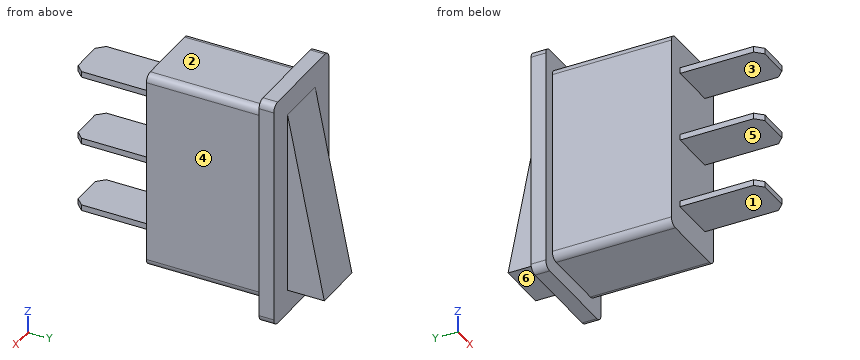
from build123d import *

# Parameters (mm, degrees)
SKIZZE1_W                            = 14
SKIZZE1_H                            = 31.5
AUFSATZ_LINEAR_AUSTRAGEN1_DEPTH      = 2
VERRUNDUNG1_R                        = 1
SKIZZE2_W                            = 10.7
SKIZZE2_H                            = 27.2
AUFSATZ_LINEAR_AUSTRAGEN2_DEPTH      = 16.2
VERRUNDUNG2_R                        = 1
SKIZZE3_W                            = 6.3
SKIZZE3_H                            = 0.8
AUFSATZ_LINEAR_AUSTRAGEN3_DEPTH      = 11
LINEARES_MUSTER1_COUNT               = 2
LINEARES_MUSTER1_PITCH               = 9.5
LINEARES_MUSTER1_COL_COUNT           = 2
LINEARES_MUSTER1_COL_PITCH           = 9.5
SCHNITT_LINEAR_AUSTRAGEN1_DEPTH      = 40.921955112
AUFSATZ_LINEAR_AUSTRAGEN4_DEPTH      = 3.5
AUFSATZ_LINEAR_AUSTRAGEN4_DEPTH_BACK = 3.5


with BuildPart() as part:
    # Skizze1 → Aufsatz-Linear austragen1 (new body)
    with BuildSketch(Plane(origin=(0, 0, 0), x_dir=(1, 0, 0), z_dir=(0, 1, 0))):
        with Locations((7, 15.75)):
            Rectangle(SKIZZE1_W, SKIZZE1_H)
    extrude(amount=AUFSATZ_LINEAR_AUSTRAGEN1_DEPTH)

    # Verrundung1
    verrundung1_edges = [part.edges().sort_by_distance(p)[0] for p in [
        (0, 1, -31.5),
        (14, 1, -31.5),
        (14, 1, 0),
        (0, 1, 0),
    ]]
    fillet(verrundung1_edges, radius=VERRUNDUNG1_R)

    # Skizze2 → Aufsatz-Linear austragen2 (add)
    with BuildSketch(Plane.XZ):
        with Locations((7, -15.75)):
            Rectangle(SKIZZE2_W, SKIZZE2_H)
    extrude(amount=AUFSATZ_LINEAR_AUSTRAGEN2_DEPTH)

    # Verrundung2
    verrundung2_edges = [part.edges().sort_by_distance(p)[0] for p in [
        (12.35, -8.1, -29.35),
        (12.35, -8.1, -2.15),
        (1.65, -8.1, -2.15),
        (1.65, -8.1, -29.35),
    ]]
    fillet(verrundung2_edges, radius=VERRUNDUNG2_R)

    # Skizze3 → Aufsatz-Linear austragen3 (add)
    with BuildSketch(Plane.XZ.offset(16.2)):
        with Locations((7, -15.75)):
            Rectangle(SKIZZE3_W, SKIZZE3_H)
    aufsatz_linear_austragen3 = extrude(amount=AUFSATZ_LINEAR_AUSTRAGEN3_DEPTH)

    # Lineares Muster1: Aufsatz-Linear austragen3 ×2
    with Locations(*[(0, 0, -i * LINEARES_MUSTER1_PITCH) for i in range(1, LINEARES_MUSTER1_COUNT)]):
        add(aufsatz_linear_austragen3)

    # Lineares Muster1 col: Aufsatz-Linear austragen3 ×2
    with Locations(*[(0, 0, i * LINEARES_MUSTER1_COL_PITCH) for i in range(1, LINEARES_MUSTER1_COL_COUNT)]):
        add(aufsatz_linear_austragen3)

    # Skizze4 → Schnitt-Linear austragen1 (cut, through all)
    with BuildSketch(Plane.XY.offset(-5.85)):
        Polygon((3.85, -26.2), (3.85, -27.2), (4.85, -27.2), align=None)
        Polygon((9.15, -27.2), (10.15, -26.2), (10.15, -27.2), align=None)
    extrude(amount=-SCHNITT_LINEAR_AUSTRAGEN1_DEPTH, mode=Mode.SUBTRACT)

    # Skizze5 → Aufsatz-Linear austragen4 (add, two sides: drawn at the far end of the back side and taken through both)
    with BuildSketch(Plane(origin=(7, 0, 0), x_dir=(0, 0, -1), z_dir=(1, 0, 0)).offset(-AUFSATZ_LINEAR_AUSTRAGEN4_DEPTH_BACK)):
        Polygon((3.25, 2), (28.25, 7), (28.25, 2), align=None)
    extrude(amount=AUFSATZ_LINEAR_AUSTRAGEN4_DEPTH + AUFSATZ_LINEAR_AUSTRAGEN4_DEPTH_BACK)


solid = part.part
Source: CAD feature listing. Evaluate the final solid. Frame: model axes, mm. Face numbers are marked on the shaded views. A direction names the side the tool comes from. Round coordinates to 2 decimals unless told otherwise and drop trailing zeros. Loops run counter-clockwise (first coordinate to the right, second up) from the corner with the lowest first, then second, coordinate; pieces in that order, holes last.
Q1. Access query for the marked faces 1, 2 and 3. Directions: +Z, -Z, +X, -X, +Y, -Y. A direction counts if a zero-diameter tool reaches every point of the face in a straight line with its end or side. Return the directions, or none.
Q2. Section C-C, the plane y = -13.5. Return loops of the section in (x, z), plus the area to 3 significant figures.
Q3. Section D-D, the plane x = 5.75. Return loops of the section in (y, z).
Q4. Section B-B, the plane z = -18. Return loops of the section in (x, y), plus the area to 3 significant figures.
Q5. Mould query, pull axis Z, two halves, no side actions, for the marked faces 4, 5 and 6. Classes: pulls with the +Z half, pulls with the -Z half, needs draft (parallel to the pull), parting line crosses it, or undercut.
Q6. First-contact query: P1, Ø3, axis at x = 11, y = -17, coming from the +Z side; P2, Ø1.5, axis at x = 5, y = -9, coming from the -Z side; P3, Ø7, axis at x = 7, y = -21.5, coming from the -Z side; P4, Ø5, axis at x = 5, y = -1.5, coming from the -Z side. Flat tips, straight axial feed; report the tip coordinate or a pass-through.
Q7. Ray query, line 1 (Z direction, x = 6.5, y = -26); line 2 (Y direction, x = 2.75, z = -19); line 3 (X direction, y = -1.5, z = -6.5). Return the intervals inside material, ascending.
Q8. Section A-A, the plane y = -20.5. Return loops of the section in (x, z), plus the area to 3 significant figures.
Solutions:
1. face 1: -Z, +X, -X, -Y
1. face 2: +Z, +X, -X, -Y
1. face 3: +X, -X, -Y
2. outline: (1.65, -28.35) arc R1 ccw to (2.65, -29.35) - (11.35, -29.35) arc R1 ccw to (12.35, -28.35) - (12.35, -3.15) arc R1 ccw to (11.35, -2.15) - (2.65, -2.15) arc R1 ccw to (1.65, -3.15) - close
2. area: 290 mm2
3. outline: (-27.2, -25.65) - (-16.2, -25.65) - (-16.2, -29.35) - (0, -29.35) - (0, -31.5) - (2, -31.5) - (2, -28.25) - (7, -28.25) - (2, -3.25) - (2, 0) - (0, 0) - (0, -2.15) - (-16.2, -2.15) - (-16.2, -5.85) - (-27.2, -5.85) - (-27.2, -6.65) - (-16.2, -6.65) - (-16.2, -15.35) - (-27.2, -15.35) - (-27.2, -16.15) - (-16.2, -16.15) - (-16.2, -24.85) - (-27.2, -24.85) - close
4. outline: (0, 0) - (1.65, 0) - (1.65, -16.2) - (12.35, -16.2) - (12.35, 0) - (14, 0) - (14, 2) - (10.5, 2) - (10.5, 4.95) - (3.5, 4.95) - (3.5, 2) - (0, 2) - close
4. area: 222 mm2
5. face 4: needs draft
5. face 5: undercut
5. face 6: pulls with the -Z half
6. P1: stops at z = -2.15
6. P2: stops at z = -29.35
6. P3: stops at z = -25.65
6. P4: stops at z = -31.5
7. line 1: z = -25.65 to -24.85, -16.15 to -15.35, -6.65 to -5.85
7. line 2: y = -16.2 to 2
7. line 3: x = 1.65 to 12.35
8. outline: (3.85, -25.65) - (10.15, -25.65) - (10.15, -24.85) - (3.85, -24.85) - close; (3.85, -16.15) - (10.15, -16.15) - (10.15, -15.35) - (3.85, -15.35) - close; (3.85, -6.65) - (10.15, -6.65) - (10.15, -5.85) - (3.85, -5.85) - close
8. area: 15.1 mm2
